Read the model definition and answer for the solid it produces. Units are mm, in the model's axes. A direction names the side the tool comes from. Round coordinates to 2 decimals unless told otherwise and drop trailing zeros. Order: outer loops, then holes, each group sorted by start corner. A loop starts at its lowest first (then second) coordinate and runs counter-clockwise, first axis right, second up.
from build123d import *

# Parameters (mm, degrees)
BOSS_EXTRUDE1_DEPTH = 1.27
SKETCH2_R           = 2.0955
CUT_EXTRUDE1_DEPTH  = 67.984946971
CHAMFER1_SIZE       = 1.27


with BuildPart() as part:
    # Sketch1 → Boss-Extrude1 (new body)
    with BuildSketch(Plane.XY):
        with BuildLine():
            Line((41.346078307, 38.223115267), (41.346078307, 29.226984353))
            Line((41.346078307, 29.226984353), (42.327409422, 30.115984353))
            ThreePointArc((42.327409422, 30.115984353), (43.232863688, 30.154994662), (43.809226811, 29.455584353))
            Line((43.809226811, 29.455584353), (45.345946242, 13.605984353))
            ThreePointArc((45.345946242, 13.605984353), (47.617277769, 15.604942198), (48.616615569, 18.460831434))
            Line((48.616615569, 18.460831434), (49.637067337, 31.131984353))
            ThreePointArc((49.637067337, 31.131984353), (50.585693925, 31.847551598), (50.544785665, 33.035093345))
            ThreePointArc((50.544785665, 33.035093345), (49.545142222, 37.023211652), (50.724981076, 40.961784353))
            Line((50.724981076, 40.961784353), (50.724981076, 41.545984353))
            ThreePointArc((50.724981076, 41.545984353), (46.883278307, 43.730384353), (43.041575539, 41.545984353))
            Line((43.041575539, 41.545984353), (43.041575539, 38.223115267))
            Line((43.041575539, 38.223115267), (41.346078307, 38.223115267))
        make_face()
    extrude(amount=BOSS_EXTRUDE1_DEPTH)

    # Sketch2 → Cut-Extrude1 (cut, through all)
    with BuildSketch(Plane.XY.offset(1.27)):
        with Locations((46.883278307, 39.259984353)):
            Circle(SKETCH2_R)
    extrude(amount=-CUT_EXTRUDE1_DEPTH, mode=Mode.SUBTRACT)

    # Chamfer1
    chamfer1_edges = [part.edges().sort_by_distance(p)[0] for p in [
        (47.617277769, 15.604942198, 1.27),
        (49.126841453, 24.796407893, 1.27),
    ]]
    chamfer(chamfer1_edges, length=CHAMFER1_SIZE - 0.0001)  # a hair under: the kernel refuses the full size


solid = part.part
Q1. A cutting plane is placed at B-B, the plane z = 0.25. Give the vertices of the cut face in (x, y).
Outcome:
outline: (41.35, 29.23) - (42.33, 30.12) arc R1.02 cw to (43.81, 29.46) - (45.32, 13.87) arc R5.72 ccw to (48.37, 18.48) - (49.38, 31.11) arc R1.29 ccw to (50.54, 33.04) arc R7.75 cw to (50.72, 40.96) - (50.72, 41.55) arc R4.47 ccw to (43.04, 41.55) - (43.04, 38.22) - (41.35, 38.22) - close; hole circle Ø4.19 at (46.88, 39.26)
Q2. A cutting plane is placed at D-D, the plane x = 42. Give the vertices of the cut face in (y, z), plus the area to 3 significant figures.
Outcome:
outline: (29.82, 0) - (38.22, 0) - (38.22, 1.27) - (29.82, 1.27) - close
area: 10.7 mm2
Q3. A cutting plane is placed at A-A, the plane y = 37.5. Give the vertices of the cut face in (x, z).
Outcome:
outline: (41.35, 0) - (45.75, 0) - (45.75, 1.27) - (41.35, 1.27) - close; (48.02, 0) - (49.57, 0) - (49.57, 1.27) - (48.02, 1.27) - close
Q4. For a pull along X with two mould halves and no side action, classify faces 4 (the face through (43.042, 40, 1)), 5 (the face through (46.96, 16.003, 0.767)), 6 (the face through (43.22, 30.16, 0.63)) as released by +X, released by -X, zero draft, split by the parting line, or undercut.
Outcome:
face 4: released by -X
face 5: released by +X
face 6: undercut
Q5. Straight lines are drawn through the part: probe 1 along X at (y, z) = (37, 0.95); probe 2 along X at (y, z) = (37.5, 0.9); probe 3 along X at (y, z) = (39.5, 1.2). For each, find the intervals that lie inside material, in ascending order.
Outcome:
probe 1: x = 41.35 to 49.54
probe 2: x = 41.35 to 45.75, 48.02 to 49.57
probe 3: x = 43.04 to 44.8, 48.96 to 50.01
Q6. For faces 1 (the face through (42, 38.223, 1)), 2 (the face through (41.83, 29.665, 0.626)), 3 (the face through (41.346, 34, 1)), determine the directions among +Z, -Z, +X, -X, +Y, -Y from which every point of the face is accessible in a straight line to the end or side of a thin tool.
Outcome:
face 1: +Z, -Z, -X, +Y
face 2: +Z, -Z, -Y
face 3: +Z, -Z, -X, +Y, -Y
